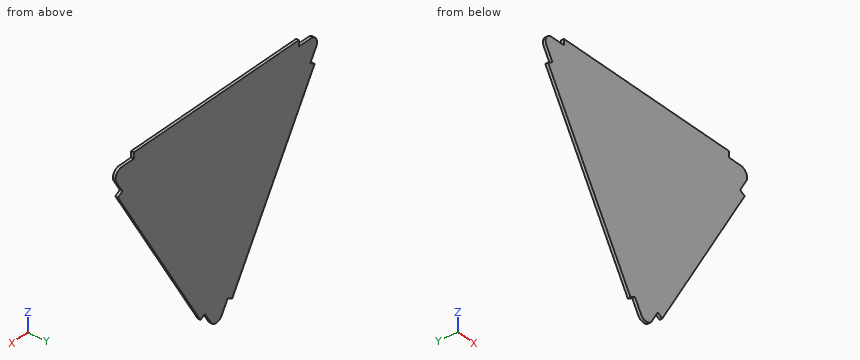
```python
from build123d import *

# Parameters (mm, degrees)
BOSS_EXTRUDE2_DEPTH = 2
CUT_EXTRUDE1_DEPTH  = 5
CIRPATTERN1_COUNT   = 3


with BuildPart() as part:
    # Sketch2 → Boss-Extrude2 (new body)
    with BuildSketch(Plane(origin=(0, 0, 0), x_dir=(1, 0, 0), z_dir=(0, 1, 0))):
        with BuildLine():
            Line((91.339745962, -42.735026919), (8.660254038, 100.470053838))
            ThreePointArc((8.660254038, 100.470053838), (0, 105.470053838), (-8.660254038, 100.470053838))
            Line((-8.660254038, 100.470053838), (-91.339745962, -42.735026919))
            ThreePointArc((-91.339745962, -42.735026919), (-91.339745962, -52.735026919), (-82.679491924, -57.735026919))
            Line((-82.679491924, -57.735026919), (82.679491924, -57.735026919))
            ThreePointArc((82.679491924, -57.735026919), (91.339745962, -52.735026919), (91.339745962, -42.735026919))
        make_face()
        with BuildLine():
            ThreePointArc((5.196152423, 98.470053838), (0, 101.470053838), (-5.196152423, 98.470053838))
            Line((-5.196152423, 98.470053838), (-87.875644347, -44.735026919))
            ThreePointArc((-87.875644347, -44.735026919), (-87.875644347, -50.735026919), (-82.679491924, -53.735026919))
            Line((-82.679491924, -53.735026919), (82.679491924, -53.735026919))
            ThreePointArc((82.679491924, -53.735026919), (87.875644347, -50.735026919), (87.875644347, -44.735026919))
            Line((87.875644347, -44.735026919), (5.196152423, 98.470053838))
        make_face(mode=Mode.SUBTRACT)
        with BuildLine():
            Line((87.875644347, -44.735026919), (5.196152423, 98.470053838))
            ThreePointArc((5.196152423, 98.470053838), (0, 101.470053838), (-5.196152423, 98.470053838))
            Line((-5.196152423, 98.470053838), (-87.875644347, -44.735026919))
            ThreePointArc((-87.875644347, -44.735026919), (-87.875644347, -50.735026919), (-82.679491924, -53.735026919))
            Line((-82.679491924, -53.735026919), (82.679491924, -53.735026919))
            ThreePointArc((82.679491924, -53.735026919), (87.875644347, -50.735026919), (87.875644347, -44.735026919))
        make_face()
    extrude(amount=BOSS_EXTRUDE2_DEPTH)

    # Sketch6 → Cut-Extrude1 (cut)
    with BuildSketch(Plane(origin=(0, 2, 0), x_dir=(1, 0, 0), z_dir=(0, 1, 0))):
        with BuildLine():
            Line((-8.660254038, 100.470053838), (-13.660254038, 91.8097998))
            Line((-13.660254038, 91.8097998), (-13.910254038, 91.376787098))
            Line((-13.910254038, 91.376787098), (-10.013139721, 89.126787098))
            Line((-10.013139721, 89.126787098), (-4.763139721, 98.220053838))
            ThreePointArc((-4.763139721, 98.220053838), (-2.75, 100.233193559), (0, 100.970053838))
            Line((0, 100.970053838), (0, 101.470053838))
            Line((0, 101.470053838), (0, 105.470053838))
            ThreePointArc((0, 105.470053838), (-5, 104.130307876), (-8.660254038, 100.470053838))
        make_face()
        with BuildLine():
            Line((-91.339745962, -42.735026919), (-86.339745962, -34.074772881))
            Line((-86.339745962, -34.074772881), (-86.089745962, -33.641760179))
            Line((-86.089745962, -33.641760179), (-82.192631645, -35.891760179))
            Line((-82.192631645, -35.891760179), (-87.442631645, -44.985026919))
            ThreePointArc((-87.442631645, -44.985026919), (-88.173795368, -47.985286122), (-87.172908415, -50.906652408))
            Line((-87.172908415, -50.906652408), (-91.089745962, -53.168039621))
            Line((-91.089745962, -53.168039621), (-91.339745962, -52.735026919))
            ThreePointArc((-91.339745962, -52.735026919), (-92.679491924, -47.735026919), (-91.339745962, -42.735026919))
        make_face()
    cut_extrude1 = extrude(amount=-CUT_EXTRUDE1_DEPTH, mode=Mode.SUBTRACT)

    # CirPattern1: Cut-Extrude1 ×3 about axis
    cirpattern1_axis = Axis((0, 0, 0), (0, 1, 0))
    for i in range(1, CIRPATTERN1_COUNT):
        add(cut_extrude1.rotate(cirpattern1_axis, i * 360 / CIRPATTERN1_COUNT), mode=Mode.SUBTRACT)


solid = part.part
```
Part model, mm, in its own coordinate system. Round coordinates to 2 decimals unless told otherwise and drop trailing zeros. Write each loop counter-clockwise with the first axis right and the second up, starting at its lowest first coordinate (ties: lowest second). Pieces come first, ordered by that corner, then holes.
Item 1: Cut at C-C, the plane x = 37. Give the cut face in (y, z).
Results:
outline: (0, -51.38) - (2, -51.38) - (2, 57.74) - (0, 57.74) - close
Item 2: Drop flat-ended pins along their axis: pin 1 Ø0.6 at (x, y) = (79.5, 1.5) entering from +Z (3 decimals); pin 2 Ø3 at (x, z) = (47, -38) entering from -Y. Give the stop position or say it passes through.
Results:
pin 1: stops at z = 53.235
pin 2: passes through
Item 3: Cut at B-B, the plane z = -64.5. Give the cut face in (x, y), plus the area to 3 significant figures.
Results:
outline: (-29.43, 0) - (29.43, 0) - (29.43, 2) - (-29.43, 2) - close
area: 118 mm2
Item 4: Probe L1, parallel to X at y = 0.4, z = -89.5; L2, parallel to Z at x = 0.5, y = 1.35; L3, parallel to Z at x = 17, y = 1.55. List the from-to ranges inside material, lowest first.
Results:
L1: x = -14.99 to -10.66, -9.8 to 9.8, 10.66 to 14.99
L2: z = -100.95 to 57.74
L3: z = -86.03 to 57.74
Item 5: Cut at A-A, the plane y = 1.25. Give the cut face in (x, z), plus the area to 3 significant figures.
Results:
outline: (-87.44, 44.99) - (-82.19, 35.89) - (-86.09, 33.64) - (-13.91, -91.38) - (-10.01, -89.13) - (-4.76, -98.22) arc R5.5 ccw to (4.76, -98.22) - (10.01, -89.13) - (13.91, -91.38) - (86.09, 33.64) - (82.19, 35.89) - (87.44, 44.99) arc R5.5 ccw to (82.68, 53.24) - (72.18, 53.24) - (72.18, 57.74) - (-72.18, 57.74) - (-72.18, 53.24) - (-82.68, 53.24) arc R5.5 ccw to start
area: 16,600 mm2
